For this review, take the finished solid that the model builds, in its own axes (mm). Face numbers are marked on the shaded views. Give positions to 0.01 mm unless a question says otherwise; leave off trailing zeros. Write each loop counter-clockwise with the first axis right and the second up, starting at its lowest first coordinate (ties: lowest second). Pieces come first, ordered by that corner, then holes.
1) Wall thickness on line 1 along Y through (x, z) = (7.25, -3); line 2 along Y through (x, z) = (2, 0.5); line 3 along Z through (x, y) = (8.75, -4.5): over which ranges is each line inside the solid? List them lowest first.
2) We need section A-A on y = 0. Give the boundary of the cut face in (x, z), and give its area (3 significant figures).
3) Draft analysis for pull direction Y (two halves, no side actions). For the marked faces 1, 2 and 3, state which applies: pulls with the +Y half, pulls with the -Y half, needs draft (parallel to the pull), parting line crosses it, or undercut.
4) We need section B-B on x = 5.5. Give the boundary of the cut face in (y, z).
5) For P1, Ø1, axis at y = -2, z = -7, coming from the -X side; P2, Ø6, axis at x = 8, z = 5.5, coming from the -Y side; P3, Ø8, axis at y = 0, z = 0, coming from the -X side, all flat-tipped, find the tip position at first contact; note any pin that passes through.
from build123d import *

# Parameters (mm, degrees)
SKETCH_2_OUTSIDE_W  = 30.08
SKETCH_2_OUTSIDE_H  = 30.08
CUT_EXTRUDE_1_DEPTH = 19.706148722


with BuildPart() as part:
    # Эскиз1 → Повернуть1 (revolve)
    with BuildSketch(Plane.XY, mode=Mode.PRIVATE) as revolve_1_sk:
        Polygon((0.9, 5.1), (9.9, 5.1), (10.8, 6), (10.8, 8.25), (9.327756814, 10.8), (1.472243186, 10.8), (0, 8.25), (0, 6), align=None)
    revolve(revolve_1_sk.sketch.rotate(Axis((0, 0, 0), (1, 0, 0)), 90), axis=Axis((0, 0, 0), (1, 0, 0)))

    # Эскиз2 outside → Вырез-Вытянуть1 (cut, through all)
    with BuildSketch(Plane.ZY):
        Rectangle(SKETCH_2_OUTSIDE_W, SKETCH_2_OUTSIDE_H)
        Polygon((0, 10.392304845), (-9, 5.196152423), (-9, -5.196152423), (0, -10.392304845), (9, -5.196152423), (9, 5.196152423), align=None, mode=Mode.SUBTRACT)
    extrude(amount=-CUT_EXTRUDE_1_DEPTH, mode=Mode.SUBTRACT)


solid = part.part
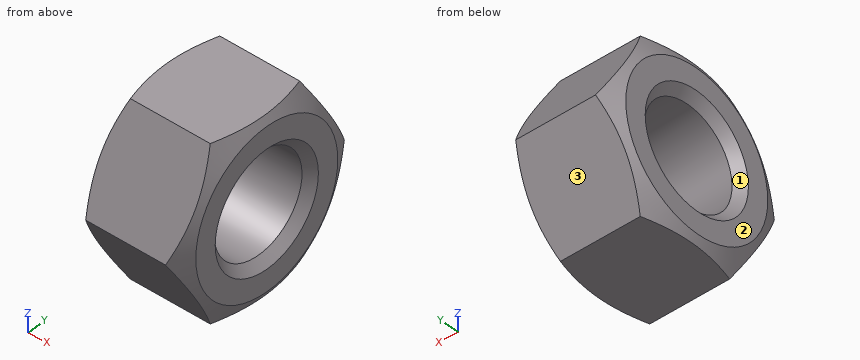
Results list:
1. line 1: y = -8.66 to -4.12, 4.12 to 8.66
1. line 2: y = -10.1 to -5.08, 5.08 to 10.1
1. line 3: z = -9 to -2.4, 2.4 to 9
2. outline: (0, -8.25) - (0.43, -9) - (10.37, -9) - (10.8, -8.25) - (10.8, -6) - (9.9, -5.1) - (0.9, -5.1) - (0, -6) - close; (0, 6) - (0.9, 5.1) - (9.9, 5.1) - (10.8, 6) - (10.8, 8.25) - (10.37, 9) - (0.43, 9) - (0, 8.25) - close
2. area: 82.0 mm2
3. face 1: undercut
3. face 2: needs draft
3. face 3: pulls with the +Y half
4. outline: (-10.39, 0) - (-5.2, -9) - (5.2, -9) - (10.39, 0) - (5.2, 9) - (-5.2, 9) - close; hole circle Ø10.2 at (0, 0)
5. P1: stops at x = 0
5. P2: stops at y = -8.95
5. P3: passes through
